from build123d import *

# Parameters (mm, degrees)
F0_W     = 50
F0_H     = 50
F0_R     = 7.75
F1_DEPTH = 20
F2_R     = 17.6
F2_R_2   = 7.75
F3_DEPTH = 8
F4_R     = 12.5
F4_R_2   = 7.75
F5_DEPTH = 5


with BuildPart() as f1:
    # F0 (on Top) → F1 (new body)
    with BuildSketch(Plane.XY):
        Rectangle(F0_W, F0_H)
        Circle(F0_R, mode=Mode.SUBTRACT)
    extrude(amount=F1_DEPTH)

    # F2 (on face) → F3 (cut)
    with BuildSketch(Plane.XY.offset(20)):
        Circle(F2_R)
        Circle(F2_R_2, mode=Mode.SUBTRACT)
    extrude(amount=-F3_DEPTH, mode=Mode.SUBTRACT)

    # F4 (on face) → F5 (cut)
    with BuildSketch(Plane(origin=(0, 0, 0), x_dir=(1, 0, 0), z_dir=(0, 0, -1))):
        Circle(F4_R)
        Circle(F4_R_2, mode=Mode.SUBTRACT)
    extrude(amount=-F5_DEPTH, mode=Mode.SUBTRACT)


solid = f1.part
Check sheet for the modelled part. Datum: model origin and axes. Units: mm. A direction names the side the tool comes from. Round coordinates to 2 decimals unless told otherwise and drop trailing zeros. Write each loop counter-clockwise with the first axis right and the second up, starting at its lowest first coordinate (ties: lowest second). Pieces come first, ordered by that corner, then holes. Notation, with made-up numbers: (55, -22.75) -> (66, -22.75) arc R13 cw to (66, 0.25) -> close; hole circle Ø8 at (57, 50). An arc over 180 degrees is marked (long way). Answer as CSV lines item,"result". Start each with the question number.
1) Release check for a two-part mould opening along X. For faces 1 (the flat face through (8, -4, 12)), 2 (the flat face through (-25, 0, 10)), 3 (the flat face through (-5.9, 11.5, 0)) record: pulls with the +X half, pulls with the -X half, needs draft (parallel to the pull), parting line crosses it, or undercut.
2) Section check A-A on x = 0. Enter the section's corners in (y, z).
3) Material ranges on line 1 (Y direction, x = 0, z = 10.5); line 2 (X direction, y = 0, z = 1.55), recorded low to high. Write a range as from..to.
4) Tool access check on faces 4 (the flat face through (25, 0, 10)), 5 (the cylindrical face through (11.923, -3.755, 2.465)), 6 (the cylindrical face through (16.787, 5.287, 16.056)). Record the directions out of +Z, -Z, +X, -X, +Y, -Y that give a thin tool (end or side, any length) a straight path to the whole face; none if there is none.
5) Section check D-D on x = 14.5. Enter the section's corners in (y, z).
6) Go/stop test with flat-tipped pins: P1, Ø12.5, axis at x = 5, y = -2, coming from the -Z side; P2, Ø4, axis at x = 17, y = 0.5, coming from the +Z side; P3, Ø10.5, axis at x = 5, y = -2.5, coming from the +Z side. Record where each tip stops, or that it passes through.
7) Section check C-C on z = 14.25. Enter the section's corners in (x, y).
Found:
1,face 1,"undercut"
1,face 2,"pulls with the -X half"
1,face 3,"needs draft"
2,outline,"(-25, 0) -> (-12.5, 0) -> (-12.5, 5) -> (-7.75, 5) -> (-7.75, 12) -> (-17.6, 12) -> (-17.6, 20) -> (-25, 20) -> close; (7.75, 5) -> (12.5, 5) -> (12.5, 0) -> (25, 0) -> (25, 20) -> (17.6, 20) -> (17.6, 12) -> (7.75, 12) -> close"
3,line 1,"y = -25..-7.75, 7.75..25"
3,line 2,"x = -25..-12.5, 12.5..25"
4,face 4,"+Z, -Z, +X, +Y, -Y"
4,face 5,"-Z"
4,face 6,"+Z"
5,outline,"(-25, 0) -> (25, 0) -> (25, 20) -> (9.98, 20) -> (9.98, 12) -> (-9.98, 12) -> (-9.98, 20) -> (-25, 20) -> close"
6,P1,"stops at z = 5"
6,P2,"stops at z = 20"
6,P3,"stops at z = 12"
7,outline,"(-25, -25) -> (25, -25) -> (25, 25) -> (-25, 25) -> close; hole circle Ø35.2 at (0, 0)"
